The model under review builds one solid part; all positions refer to its coordinate system, in mm. A direction names the side the tool comes from. Coordinates: 2 decimals unless noted, no trailing zeros. Loops run counter-clockwise (first coordinate to the right, second up) from the corner with the lowest first, then second, coordinate; pieces in that order, holes last. Notation, with made-up numbers: M -1,-1.5 L 25,-1.5 A12 ccw 25,11.5 Z; hole C 8.5,-28.5 d11. An arc over 180 degrees is marked long. Use CSV: the item, a comma, the result in double quotes. Start each with the question number.
1. Tool access review of faces 5 (the flat face through (-12, 1, 0)), 6 (the flat face through (-3.25, -24, 2)): name each direction out of +Z, -Z, +X, -X, +Y, -Y from which nothing blocks a thin tool from reaching the whole face with its end or side.
2. For L1, parallel to Y at x = 8.5, z = 3.05; L2, parallel to X at y = 45.5, z = 0.3; L3, parallel to X at y = 43, z = 3.6, list the stretches that pass through material, from the lowest coordinate up.
3. Add section C-C, the plane z = 1.35. State how many separate pieces and enclosed holes the cut face has, then the cut area to 3 significant figures.
4. Add section D-D, the plane y = 35.5. Write out the cut boundary in (x, z), then the cut area to 3 significant figures.
5. Add section A-A, the plane y = 17.5. Write out the cut boundary in (x, z), then the cut area to 3 significant figures.
6. Add section B-B, the plane y = 70.3. Write out the cut boundary in (x, z).
7. Clearance check with a flat-ended pin moving along its axis: P1, Ø10, axis at x = 11, y = -40, coming from the -Z side. State where the tip first meets the part, or that it passes through.
8. Draft analysis for pull direction X (two halves, no side actions). For faces 1 (the flat face through (18.1, 6, 2)), 2 (the cylindrical face through (-1.575, -36.303, 1.977)), 3 (the flat face through (-18.1, 5, 2)), 4 (the cylindrical face through (13.621, -26.436, 2.028)), state which applies: +X half, -X half, draft (parallel to the pull), parting line (faces both ways), or undercut.
from build123d import *

# Parameters (mm, degrees)
SKETCH1_R          = 12.1
SKETCH1_W          = 20.2
SKETCH1_H          = 40.2
BASE_PLATE_DEPTH   = 4
FILLET1_R          = 1
FILLET2_R          = 2
SKETCH2_R          = 1.7
CUT_EXTRUDE1_DEPTH = 78.256779638
SKETCH5_W          = 6.5
SKETCH5_H          = 7.3
CUT_EXTRUDE3_DEPTH = 78.256779638
FILLET4_R          = 1
FILLET5_R          = 0.35


with BuildPart() as part:
    # Sketch1 → Base Plate (new body)
    with BuildSketch(Plane.XY):
        with BuildLine():
            Line((-18.1, -62), (-18.1, 75))
            Line((-18.1, 75), (18.1, 75))
            Line((18.1, 75), (18.1, -62))
            ThreePointArc((18.1, -62), (14.292388155, -71.192388155), (5.1, -75))
            Line((5.1, -75), (-5.1, -75))
            ThreePointArc((-5.1, -75), (-14.292388155, -71.192388155), (-18.1, -62))
        make_face()
        with Locations((0, -48.3)):
            Circle(SKETCH1_R, mode=Mode.SUBTRACT)
        Polygon((-10.1, 28.1), (4.1, 28.1), (-10.1, 67), align=None, mode=Mode.SUBTRACT)
        Rectangle(SKETCH1_W, SKETCH1_H, mode=Mode.SUBTRACT)
        Polygon((10.1, 67), (-4.1, 67), (10.1, 28.1), align=None, mode=Mode.SUBTRACT)
    extrude(amount=BASE_PLATE_DEPTH)

    # Fillet1
    fillet1_edges = [part.edges().sort_by_distance(p)[0] for p in [
        (10.1, 28.1, 2),
        (10.1, 67, 2),
        (-4.1, 67, 2),
        (-10.1, 67, 2),
        (-10.1, 28.1, 2),
        (4.1, 28.1, 2),
    ]]
    fillet(fillet1_edges, radius=FILLET1_R)

    # Fillet2
    fillet2_edges = [part.edges().sort_by_distance(p)[0] for p in [
        (-18.1, 75, 2),
        (18.1, 75, 2),
    ]]
    fillet(fillet2_edges, radius=FILLET2_R)

    # Sketch2 → Cut-Extrude1 (cut, through all)
    with BuildSketch(Plane.XY.offset(4)):
        with Locations((5, 24.75)):
            Circle(SKETCH2_R)
        with Locations((-5, 24.75)):
            Circle(SKETCH2_R)
        with Locations(Location((-5, -24.75, 0), (0, 0, 180))):
            Circle(SKETCH2_R)
        with Locations(Location((5, -24.75, 0), (0, 0, 180))):
            Circle(SKETCH2_R)
        with Locations((13.4, 24.75)):
            Circle(SKETCH2_R)
        with Locations(Location((-13.4, 24.75, 0), (0, 0, 180))):
            Circle(SKETCH2_R)
        with Locations(Location((13.4, -24.75, 0), (0, 0, 180))):
            Circle(SKETCH2_R)
        with Locations((-13.4, -24.75)):
            Circle(SKETCH2_R)
        with Locations((13.4, 70.3)):
            Circle(SKETCH2_R)
        with Locations(Location((-13.4, 70.3, 0), (0, 0, 180))):
            Circle(SKETCH2_R)
        with Locations((0, -69.3)):
            Circle(SKETCH2_R)
    extrude(amount=-CUT_EXTRUDE1_DEPTH, mode=Mode.SUBTRACT)

    # Sketch5 → Cut-Extrude3 (cut, through all)
    with BuildSketch(Plane.XY.offset(4)):
        with Locations((0, -23.75)):
            Rectangle(SKETCH5_W, SKETCH5_H)
    extrude(amount=-CUT_EXTRUDE3_DEPTH, mode=Mode.SUBTRACT)

    # Fillet4
    fillet4_edges = [part.edges().sort_by_distance(p)[0] for p in [
        (-3.25, -27.4, 2),
        (-3.25, -20.1, 2),
        (3.25, -20.1, 2),
        (3.25, -27.4, 2),
    ]]
    fillet(fillet4_edges, radius=FILLET4_R)

    # Fillet5
    fillet5_edges = [part.edges().sort_by_distance(p)[0] for p in [
        (17.514213562, 74.414213562, 4),
        (-17.514213562, 74.414213562, 4),
        (-14.292388155, -71.192388155, 4),
        (0, -75, 4),
        (14.292388155, -71.192388155, 4),
        (-12.1, -48.3, 0),
        (-12.1, -48.3, 4),
        (18.1, 5.5, 4),
        (14.292388155, -71.192388155, 0),
        (0, -75, 0),
        (-14.292388155, -71.192388155, 0),
        (18.1, 5.5, 0),
        (-18.1, 5.5, 0),
        (-18.1, 5.5, 4),
        (0, 75, 0),
        (17.514213562, 74.414213562, 0),
        (-17.514213562, 74.414213562, 0),
        (0, 75, 4),
    ]]
    fillet(fillet5_edges, radius=FILLET5_R)


solid = part.part
Computed:
1,face 5,"-Z, +X, -X, +Y, -Y"
1,face 6,"+Z, -Z"
2,L1,"y = -74.55 to -56.91, -39.69 to -20.1, 20.1 to 32.96, 67 to 75"
2,L2,"x = -18.1 to -10.1, -2.25 to 3.75, 10.1 to 18.1"
2,L3,"x = -18.1 to -10.1, -1.34 to 4.66, 10.1 to 18.1"
3,separate pieces,"1"
3,enclosed holes,"15"
3,area,"3,390 mm^2"
4,outline,"M -18.1,0.35 A0.35 ccw -17.75,0 L -10.1,0 L -10.1,4 L -17.75,4 A0.35 ccw -18.1,3.65 Z; M 1.4,0 L 7.4,0 L 7.4,4 L 1.4,4 Z; M 10.1,0 L 17.75,0 A0.35 ccw 18.1,0.35 L 18.1,3.65 A0.35 ccw 17.75,4 L 10.1,4 Z"
4,area,"87.9 mm^2"
5,outline,"M -18.1,0.35 A0.35 ccw -17.75,0 L -10.1,0 L -10.1,4 L -17.75,4 A0.35 ccw -18.1,3.65 Z; M 10.1,0 L 17.75,0 A0.35 ccw 18.1,0.35 L 18.1,3.65 A0.35 ccw 17.75,4 L 10.1,4 Z"
5,area,"63.9 mm^2"
6,outline,"M -18.1,0.35 A0.35 ccw -17.75,0 L -15.1,0 L -15.1,4 L -17.75,4 A0.35 ccw -18.1,3.65 Z; M -11.7,0 L 11.7,0 L 11.7,4 L -11.7,4 Z; M 15.1,0 L 17.75,0 A0.35 ccw 18.1,0.35 L 18.1,3.65 A0.35 ccw 17.75,4 L 15.1,4 Z"
7,P1,"stops at z = 0"
8,face 1,"+X half"
8,face 2,"undercut"
8,face 3,"-X half"
8,face 4,"undercut"
